```python
from build123d import *

# Parameters (mm, degrees)
SKETCH1_R           = 10
SKETCH1_R_2         = 4
BOSS_EXTRUDE1_DEPTH = 8
SKETCH2_W           = 2.5
SKETCH2_H           = 11.075471698
CUT_EXTRUDE1_DEPTH  = 17.248076809
SKETCH3_R           = 1.05
CUT_EXTRUDE2_DEPTH  = 24.748684174
SKETCH4_R           = 2
CUT_EXTRUDE3_DEPTH  = 6
BOSS_EXTRUDE3_START = 6
SKETCH6_R           = 10
BOSS_EXTRUDE3_DEPTH = 6


with BuildPart() as part:
    # Sketch1 → Boss-Extrude1 (new body)
    with BuildSketch(Plane.XY):
        Circle(SKETCH1_R)
        Circle(SKETCH1_R_2, mode=Mode.SUBTRACT)
    extrude(amount=BOSS_EXTRUDE1_DEPTH)

    # Sketch2 → Cut-Extrude1 (cut, through all)
    with BuildSketch(Plane.XY.offset(8)):
        with Locations((0, 5.537735849)):
            Rectangle(SKETCH2_W, SKETCH2_H)
    extrude(amount=-CUT_EXTRUDE1_DEPTH, mode=Mode.SUBTRACT)

    # Sketch3 → Cut-Extrude2 (cut, through all)
    with BuildSketch(Plane.ZY.offset(10)):
        with Locations((4, 6.860619227)):
            Circle(SKETCH3_R)
    extrude(amount=-CUT_EXTRUDE2_DEPTH, mode=Mode.SUBTRACT)

    # Sketch4 → Cut-Extrude3 (cut)
    with BuildSketch(Plane.ZY.offset(10)):
        with Locations((4, 6.860619227)):
            Circle(SKETCH4_R)
    cut_extrude3 = extrude(amount=-CUT_EXTRUDE3_DEPTH, mode=Mode.SUBTRACT)

    # Mirror1: Cut-Extrude3 across plane
    add(cut_extrude3.mirror(Plane.ZY), mode=Mode.SUBTRACT)

    # Sketch6 → Boss-Extrude3 (add)
    with BuildSketch(Plane(origin=(0, 0, 0), x_dir=(-1, 0, 0), z_dir=(0, 0, -1)).offset(BOSS_EXTRUDE3_START)):
        Circle(SKETCH6_R)
    extrude(amount=-BOSS_EXTRUDE3_DEPTH)


solid = part.part
```
The model under review builds one solid part; all positions refer to its coordinate system, in mm. A direction names the side the tool comes from. Round coordinates to 2 decimals unless told otherwise and drop trailing zeros. Write each loop counter-clockwise with the first axis right and the second up, starting at its lowest first coordinate (ties: lowest second). Pieces come first, ordered by that corner, then holes.
(1) Wall thickness on L1, parallel to X at y = 0, z = 3; L2, parallel to X at y = 7.5, z = 2.5; L3, parallel to Y at x = -1.95, z = 4: over which ranges is each line inside the solid? List them lowest first.
(2) We need section C-C on y = 0. Give the boundary of the cut face in (x, z), and give its area (3 significant figures).
(3) We need section A-A on x = -3.5. Give the boundary of the cut face in (y, z).
(4) Insertion check: pin 1 (3 mm diameter, centred on y = 6.86, z = 4, fed in from -X); pin 2 (2 mm diameter, centred on y = -2, z = 4.5, fed in from +X); pin 3 (1 mm diameter, centred on x = -0.5, z = -2.5, fed in from +Y); pin 4 (6.5 mm diameter, centred on y = 6.86, z = 4, fed in from +X). Each pin has a flat end and moves straight along its axis. Give the tip position at first contact, or say it passes through.
(5) We need section D-D on x = 0. Give the boundary of the cut face in (y, z).
(6) We need section B-B on z = 4.25. Give the boundary of the cut face in (x, y), and give its area (3 significant figures).
(7) Machinability: for faces 5 (the cylindrical face through (-5.9, 4.9, 3.6)), 6 (the flat face through (0, 2, 0)), 7 (the flat face through (1.25, 6, 5)), 8 (the flat face through (-0.1, -4.3, 8)), 9 (the cylindrical face through (5.9, 4.9, 3.6)), which of the approach directions +Z, -Z, +X, -X, +Y, -Y give a long, thin tool a straight path to every point of the face, cutting with its end or side? Answer none if there is none.
(8) Mouldability with a two-part tool opening along X and no side actions: class faces 1 (the flat face through (-4, 6, 5)), 2 (the flat face through (4, 6, 5)), 3 (the cylindrical face through (-2.644, 7.57, 3.226)), 4 (the flat face through (-1.25, 6, 5)) as +X half, -X half, draft (parallel to the pull), parting line (faces both ways), or undercut.
Findings below:
1. L1: x = -10 to -4, 4 to 10
1. L2: x = -4 to -1.25, 1.25 to 4
1. L3: y = -9.81 to -3.49, 3.49 to 5.81, 7.91 to 9.81
2. outline: (-10, -6) - (10, -6) - (10, 8) - (4, 8) - (4, 0) - (-4, 0) - (-4, 8) - (-10, 8) - close
2. area: 216 mm2
3. outline: (-9.37, -6) - (9.37, -6) - (9.37, 8) - (1.94, 8) - (1.94, 0) - (-1.94, 0) - (-1.94, 8) - (-9.37, 8) - close; hole circle Ø2.1 at (6.86, 4)
4. pin 1: stops at x = -4
4. pin 2: stops at x = 9.95
4. pin 3: stops at y = 10
4. pin 4: stops at x = 9.33
5. outline: (-10, -6) - (10, -6) - (10, 0) - (-4, 0) - (-4, 8) - (-10, 8) - close
6. outline: (-8.73, 4.88) arc R10 ccw (long way) to (8.73, 4.88) - (4, 4.88) - (4, 5.84) - (1.25, 5.84) - (1.25, 3.8) arc R4 cw (long way) to (-1.25, 3.8) - (-1.25, 5.84) - (-4, 5.84) - (-4, 4.88) - close; (-4.67, 8.84) - (-4, 8.84) - (-4, 7.88) - (-1.25, 7.88) - (-1.25, 9.92) arc R10 ccw to start; (1.25, 7.88) - (4, 7.88) - (4, 8.84) - (4.67, 8.84) arc R10 ccw to (1.25, 9.92) - close
6. area: 213 mm2
7. face 5: -X
7. face 6: +Z
7. face 7: +Z, +Y
7. face 8: +Z, +X, -X, +Y, -Y
7. face 9: +X
8. face 1: -X half
8. face 2: +X half
8. face 3: draft
8. face 4: undercut
